from build123d import *

# Parameters (mm, degrees)
SKETCH1_R           = 2.38125
SKETCH1_R_2         = 0.75
BOSS_EXTRUDE1_DEPTH = 2


with BuildPart() as part:
    # Sketch1 → Boss-Extrude1 (new, symmetric)
    with BuildSketch(Plane(origin=(0, 0, 0), x_dir=(0, 0, -1), z_dir=(1, 0, 0))):
        with BuildLine():
            Line((-56.590412722, 6.909587278), (-51.518608779, 6.909587278))
            Line((-51.518608779, 6.909587278), (-51.518608779, 18.053715602))
            Line((-51.518608779, 18.053715602), (-16.803992093, 18.053715602))
            Line((-16.803992093, 18.053715602), (-16.803992093, 11.79733741))
            Line((-16.803992093, 11.79733741), (-43.018535026, 11.79733741))
            ThreePointArc((-43.018535026, 11.79733741), (-45.462410091, 9.353462344), (-43.018535026, 6.909587278))
            Line((-43.018535026, 6.909587278), (6.909587278, 6.909587278))
            Line((6.909587278, 6.909587278), (6.909587278, -20.222057583))
            Line((6.909587278, -20.222057583), (-43.890412722, -20.222057583))
            Line((-43.890412722, -20.222057583), (-43.890412722, -43.890412722))
            Line((-43.890412722, -43.890412722), (-56.590412722, -43.890412722))
            Line((-56.590412722, -43.890412722), (-56.590412722, 6.909587278))
        make_face()
        Circle(SKETCH1_R, mode=Mode.SUBTRACT)
        with Locations((-45.552958224, -38.810412722)):
            Circle(SKETCH1_R_2, mode=Mode.SUBTRACT)
        with Locations((-47.584958224, -38.810412722)):
            Circle(SKETCH1_R_2, mode=Mode.SUBTRACT)
        with Locations((-49.616958224, -38.810412722)):
            Circle(SKETCH1_R_2, mode=Mode.SUBTRACT)
        with Locations((-51.648958224, -38.810412722)):
            Circle(SKETCH1_R_2, mode=Mode.SUBTRACT)
        with Locations((-50.410128911, -22.137211246)):
            Circle(SKETCH1_R, mode=Mode.SUBTRACT)
        with Locations((-50.410128911, 1.079375692)):
            Circle(SKETCH1_R, mode=Mode.SUBTRACT)
        with Locations((-53.680958224, -38.810412722)):
            Circle(SKETCH1_R_2, mode=Mode.SUBTRACT)
        Polygon((-40.547855017, 3.612408172), (-21.81561352, 0.147494252), (-24.001169646, -11.668200482), (-42.733411143, -8.203286562), align=None, mode=Mode.SUBTRACT)
    extrude(amount=BOSS_EXTRUDE1_DEPTH, both=True)


solid = part.part
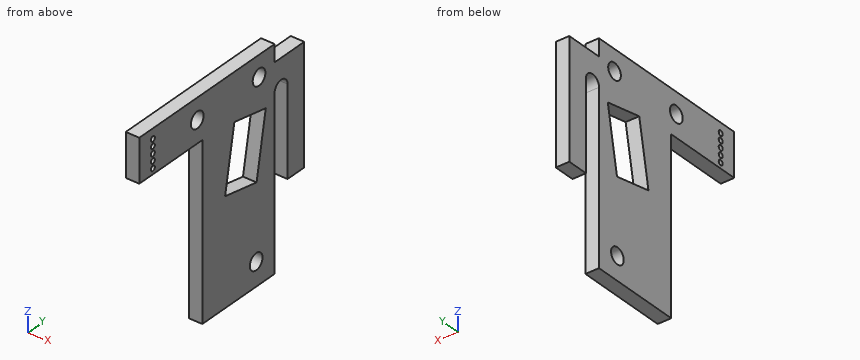
Input: part model. Units: mm. Frame: model coordinates. Coordinates: 2 decimals unless noted, no trailing zeros. Loops run counter-clockwise (first coordinate to the right, second up) from the corner with the lowest first, then second, coordinate; pieces in that order, holes last. Notation, with made-up numbers: (12, 45.25) -> (63, 45.25) arc R24 ccw to (63, 82.25) -> close; hole circle Ø11 at (37.25, 52). An arc over 180 degrees is marked (long way). Write item = value, one per line. Start each with the question number.
Item 1: Cut plane C-C, the plane z = 39. Return loops of the section in (x, y).
Item 2: Material intervals for line 1 (Y direction, x = -0.3, z = 38); line 2 (Y direction, x = 1.25, z = 34); line 3 (Y direction, x = -1.2, z = 0), sorted ascending.
Item 3: First-contact query: P1, Ø1.5, axis at x = -1, z = 10.5, coming from the +Y side; P2, Ø0.9, axis at y = -38.81, z = 49.62, coming from the +X side; P3, Ø1, axis at x = 1, y = -31.5, coming from the -Z side. Flat tips, straight axial feed; report the tip coordinate or a pass-through.
Item 4: Cut plane A-A, the plane z = 0. Return loops of the section in (x, y), plus the area to 3 significant figures.
Item 5: Cut plane D-D, the plane y = -28. Return loops of the section in (x, z), plus the area to 3 significant figures.
Item 6: Cut plane B-B, the plane x = 1. Count the separate pieces of the cut face and the enclosed holes in it, plus the area to 3 significant figures.
Ans:
q1.outline = (-2, -20.22) -> (2, -20.22) -> (2, -8.89) -> (-2, -8.89) -> close; (-2, 3.33) -> (2, 3.33) -> (2, 6.91) -> (-2, 6.91) -> close; (-2, 11.8) -> (2, 11.8) -> (2, 18.05) -> (-2, 18.05) -> close
q2.line_1 = -20.22 to -9.08, 3.14 to 6.91, 11.8 to 18.05
q2.line_2 = -20.22 to -9.82, 2.4 to 6.91, 11.8 to 18.05
q2.line_3 = -20.22 to -2.38, 2.38 to 6.91
q3.P1 = 6.91
q3.P2 = through
q3.P3 = 43.89
q4.outline = (-2, -20.22) -> (2, -20.22) -> (2, -2.38) -> (-2, -2.38) -> close; (-2, 2.38) -> (2, 2.38) -> (2, 6.91) -> (-2, 6.91) -> close
q4.area = 89.5 mm²
q5.outline = (-2, 43.89) -> (2, 43.89) -> (2, 56.59) -> (-2, 56.59) -> close
q5.area = 50.8 mm²
q6.separate_pieces = 1
q6.enclosed_holes = 9
q6.area = 1,980 mm²
